Geometry check sheet. Reference: the model listing, model coordinates, mm. A direction names the side the tool comes from. Give positions to 0.01 mm unless a question says otherwise; leave off trailing zeros. Order: outer loops, then holes, each group sorted by start corner. A loop starts at its lowest first (then second) coordinate and runs counter-clockwise, first axis right, second up. Notation, with made-up numbers: M 81,-40 L 95,-40 A20 ccw 95,-20 Z; hole C 68,-13 d4. An arc over 180 degrees is marked long. Answer as a JSON object with one key per item and string values. Group by question number.
from build123d import *

# Parameters (mm, degrees)
SKETCH1_R           = 25.4
BOSS_EXTRUDE2_DEPTH = 18.356350904
CUT_EXTRUDE1_DEPTH  = 7.62
FILLET1_R           = 7.62
CHAMFER1_SIZE       = 5.08
CHAMFER2_SIZE       = 5.08
CHAMFER3_SIZE       = 5.08
CHAMFER4_SIZE       = 5.08
CHAMFER8_SIZE       = 5.08


with BuildPart() as part:
    # Sketch1 → Boss-Extrude2 (new body)
    with BuildSketch(Plane(origin=(0, 0, 0), x_dir=(1, 0, 0), z_dir=(0, 1, 0))):
        Polygon((-342.9, 381), (-381, 381), (-381, 0), (-342.9, 0), (-38.1, 0), (0, 0), (0, 381), (-38.1, 381), align=None)
        with Locations(Location((-342.9, 38.1, 0), (0, 0, 270))):
            Circle(SKETCH1_R, mode=Mode.SUBTRACT)
        Polygon((-285.853349775, 69.85), (-311.15, 69.85), (-311.15, 95.035246339), align=None, mode=Mode.SUBTRACT)
        Polygon((-311.15, 148.798269562), (-311.15, 190.5), (-311.15, 202.561292784), (-177.851674887, 69.85), (-231.852512331, 69.85), align=None, mode=Mode.SUBTRACT)
        with Locations(Location((-38.1, 38.1, 0), (0, 0, 270))):
            Circle(SKETCH1_R, mode=Mode.SUBTRACT)
        Polygon((-311.15, 256.324316007), (-311.15, 310.08733923), (-69.85, 69.85), (-123.850837444, 69.85), align=None, mode=Mode.SUBTRACT)
        with Locations(Location((-342.9, 342.9, 0), (0, 0, 270))):
            Circle(SKETCH1_R, mode=Mode.SUBTRACT)
        Polygon((-69.85, 177.376046445), (-69.85, 123.613023223), (-257.149162556, 310.08733923), (-203.148325113, 310.08733923), align=None, mode=Mode.SUBTRACT)
        Polygon((-149.147487669, 310.08733923), (-95.146650225, 310.08733923), (-69.85, 284.902092891), (-69.85, 231.139069668), align=None, mode=Mode.SUBTRACT)
        with Locations(Location((-38.1, 342.9, 0), (0, 0, 270))):
            Circle(SKETCH1_R, mode=Mode.SUBTRACT)
    extrude(amount=BOSS_EXTRUDE2_DEPTH)

    # Sketch3 → Cut-Extrude1 (cut)
    with BuildSketch(Plane(origin=(0, 18.356350904, 0), x_dir=(1, 0, 0), z_dir=(0, 1, 0))):
        Polygon((-69.85, 177.376046445), (-69.85, 310.08733923), (-311.15, 310.08733923), (-311.15, 69.85), (-69.85, 69.85), align=None)
    extrude(amount=-CUT_EXTRUDE1_DEPTH, mode=Mode.SUBTRACT)

    # Fillet1
    fillet1_edges = [part.edges().sort_by_distance(p)[0] for p in [
        (-38.1, 18.356350904, -63.5),
        (-38.1, 18.356350904, -368.3),
        (-342.9, 18.356350904, -63.5),
        (-342.9, 18.356350904, -368.3),
    ]]
    fillet(fillet1_edges, radius=FILLET1_R)

    # Chamfer1
    chamfer1_edges = [part.edges().sort_by_distance(p)[0] for p in [
        (-69.85, 18.356350904, -189.968669615),
        (-190.5, 18.356350904, -310.08733923),
        (-190.5, 18.356350904, -69.85),
        (-311.15, 18.356350904, -189.968669615),
    ]]
    chamfer(chamfer1_edges, length=CHAMFER1_SIZE)

    # Chamfer2
    chamfer2_edges = [part.edges().sort_by_distance(p)[0] for p in [
        (-298.501674887, 10.736350904, -82.442623169),
        (-271.501256165, 10.736350904, -109.324134781),
        (-244.500837444, 10.736350904, -136.205646392),
        (-217.500418722, 10.736350904, -163.087158004),
        (-136.499162556, 10.736350904, -243.731692838),
        (-109.498743835, 10.736350904, -270.613204449),
        (-190.5, 10.736350904, -189.968669615),
        (-163.499581278, 10.736350904, -216.850181226),
        (-82.498325113, 10.736350904, -297.49471606),
    ]]
    chamfer(chamfer2_edges, length=CHAMFER2_SIZE)

    # Chamfer3
    chamfer3_edges = [part.edges().sort_by_distance(p)[0] for p in [
        (-381, 18.356350904, -190.5),
        (-190.5, 18.356350904, 0),
        (0, 18.356350904, -190.5),
        (-190.5, 18.356350904, -381),
    ]]
    chamfer(chamfer3_edges, length=CHAMFER3_SIZE - 0.0001)  # a hair under: the kernel refuses the full size

    # Chamfer4
    chamfer4_edges = [part.edges().sort_by_distance(p)[0] for p in [
        (-190.5, 0, -381),
        (0, 0, -190.5),
        (-190.5, 0, 0),
        (-381, 0, -190.5),
    ]]
    chamfer(chamfer4_edges, length=CHAMFER4_SIZE)

    # Chamfer8
    chamfer8_edges = [part.edges().sort_by_distance(p)[0] for p in [
        (-136.499162556, 0, -243.731692838),
        (-109.498743835, 0, -270.613204449),
    ]]
    chamfer(chamfer8_edges, length=CHAMFER8_SIZE)


solid = part.part
1. Access from +Z, -Z, +X, -X, +Y, -Y to the whole of each face (thin tool, end or side, straight path). Record for faces 1 (the flat face through (-162.188, 2.789, -215.545)), 2 (the flat face through (-110.676, 2.576, -268.251)), 3 (the flat face through (-272.713, 8.161, -106.997)).
2. Cross-section at C-C (z = -272). Record the cut outline in (x, y), and give its area (3 significant figures).
3. Thickness scan on line 1 along X through (y, z) = (8.75, -38.1); line 2 along X through (y, z) = (7.5, -31.5); line 3 along Z through (x, y) = (-181, 12.75). Record the ranges inside material, lowest first. Write a range as [from, to].
4. Release check for a two-part mould opening along X. For faces 4 (the flat face through (-179, 10.736, -203)), 5 (the flat face through (0, 9, -188)), 6 (the flat face through (-188, 9, -381)) record: released by +X, released by -X, zero draft, split by the parting line, or undercut.
5. Cross-section at A-A (z = -342.9). State how many separate pieces and enclosed holes the cut face has, and give its area (3 significant figures).
6. Depth check by flat-ended pin: pin 1 (4 mm diameter, centred on x = -152.5, z = -190, fed in from +Y); pin 2 (1.5 mm diameter, centred on y = 15, z = -298.5, fed in from +X); pin 3 (2 mm diameter, centred on x = -69, y = 16, fed in from +Z). Enter the tip coordinate at first touch or a pass-through.
Report:
{
 "1": {"face 1": "+Y, -Y", "face 2": "-Y", "face 3": "+Y"},
 "2": {"outline": "M -381,5.08 L -375.92,0 L -311.15,0 L -311.15,13.28 L -316.23,18.36 L -375.92,18.36 L -381,13.28 Z; M -272.89,0 L -218.89,0 L -218.89,5.66 L -226.09,10.74 L -265.69,10.74 L -272.89,5.66 Z; M -164.89,5.08 L -157.69,0 L -118.09,0 L -110.89,5.08 L -110.89,5.66 L -118.09,10.74 L -157.69,10.74 L -164.89,5.66 Z; M -69.85,0 L -5.08,0 L 0,5.08 L 0,13.28 L -5.08,18.36 L -64.77,18.36 L -69.85,13.28 Z", "area": "3,540 mm2"},
 "3": {"line 1": "x = [-381, -368.3], [-317.5, -63.5], [-12.7, 0]", "line 2": "x = [-381, -367.43], [-318.37, -62.63], [-13.57, 0]", "line 3": "z = [-381, -310.09], [-69.85, 0]"},
 "4": {"face 4": "undercut", "face 5": "released by +X", "face 6": "zero draft"},
 "5": {"separate pieces": "3", "enclosed holes": "0", "area": "5,030 mm2"},
 "6": {"pin 1": "stops at y = 10.74", "pin 2": "stops at x = -0.97", "pin 3": "stops at z = -1.72"}
}
